The drawing under review shows one solid part. Ordinate dimensions are in mm from its lowest x, y, z. Coordinates: 2 decimals unless noted, no trailing zeros. Loops run counter-clockwise (first coordinate to the right, second up) from the corner with the lowest first, then second, coordinate; pieces in that order, holes last. Notation, with made-up numbers: (11.25, -32.5) - (38.25, -32.5) arc R28 ccw to (38.25, -5.5) - close; hole circle Ø3 at (17, 53.25). An arc over 180 degrees is marked (long way). Answer as a JSON object with one key per item and string values. Group by question number.
Item 1: Clearance check with flat-ended pins moving along their axes: pin 1 (12 mm diameter, centred on x = 4.5, z = 468, fed in from -Y); pin 2 (5 mm diameter, centred on x = 11.5, z = 324, fed in from +Y); pin 3 (12 mm diameter, centred on x = 3.5, z = 515.5, fed in from -Y). State where each tip first meets the part, or that it passes through.
Item 2: We need section A-A (z = 217). Give the boundary of the cut face in (x, y), then the cut area to 3 significant figures.
Item 3: We need section B-B (x = 7.75). Give the boundary of the cut face in (y, z), then the cut area to 3 significant figures.
Item 4: To check wall thickness, follow line 1 (Y direction, x = 17.75, z = 547.5); line 2 (Y direction, x = 4, z = 516); line 3 (X direction, y = 13.5, z = 410.5). State the ranges of each line that lie inside material, in increasing order.
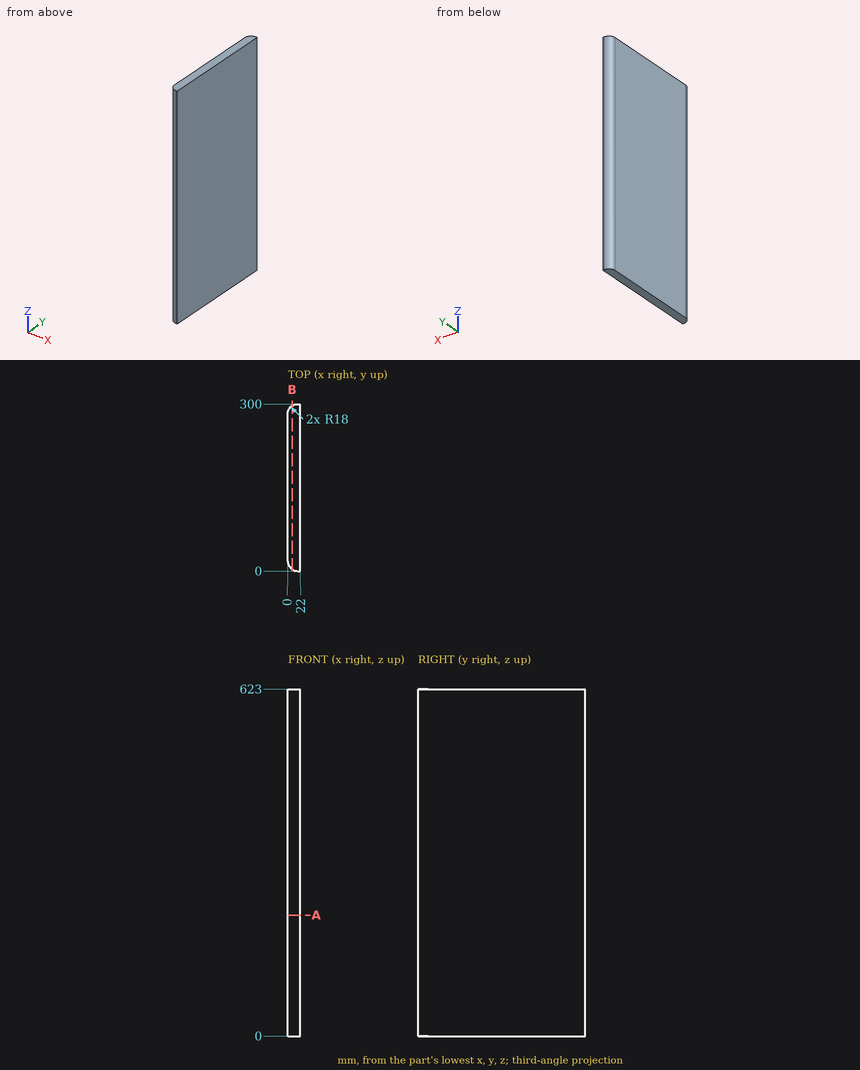
Check sheet entries:
{
 "1": {"pin 1": "stops at y = 1.64", "pin 2": "stops at y = 299.55", "pin 3": "stops at y = 2.13"},
 "2": {"outline": "(0, 18) arc R18 ccw to (18, 0) - (22, 0) - (22, 300) - (18, 300) arc R18 ccw to (0, 282) - close", "area": "6,460 mm2"},
 "3": {"outline": "(3.2, 0) - (296.8, 0) - (296.8, 623) - (3.2, 623) - close", "area": "183,000 mm2"},
 "4": {"line 1": "y = 0 to 300", "line 2": "y = 6.69 to 293.31", "line 3": "x = 0.57 to 22"}
}
